from build123d import *

# Parameters (mm, degrees)
SKETCH1_W            = 116.84
SKETCH1_H            = 86.36
BOSS_EXTRUDE2_DEPTH  = 5.08
FILLET1_R            = 12.7
SKETCH3_W            = 116.84
SKETCH3_H            = 60.96
SKETCH3_W_2          = 111.76
SKETCH3_H_2          = 55.88
BOSS_EXTRUDE3_DEPTH  = 38.1
SKETCH4_W            = 10.16
SKETCH4_H            = 10.16
BOSS_EXTRUDE5_DEPTH  = 34.29
FILLET3_R            = 5.08
SKETCH5_R            = 1.27
CUT_EXTRUDE1_DEPTH   = 34.29
CUT_EXTRUDE2_START   = -5.08
SKETCH6_W            = 198.457473549
SKETCH6_H            = 149.814535244
SKETCH6_W_2          = 116.84
SKETCH6_H_2          = 60.96
CUT_EXTRUDE2_DEPTH   = 5.08
FILLET6_R            = 5.08
CUT_EXTRUDE3_REACH   = 146.713
SKETCH7_R            = 12.7
SKETCH7_R_2          = 2.159
CUT_EXTRUDE4_REACH   = 146.713
SKETCH8_R            = 3.175
BOSS_EXTRUDE9_DEPTH  = 5.08
SKETCH14_R           = 1.27
CUT_EXTRUDE6_DEPTH   = 8.89
SKETCH21_W           = 111.76
SKETCH21_H           = 55.88
CUT_EXTRUDE7_DEPTH   = 29.21
SKETCH22_W           = 20.924478465
SKETCH22_H           = 12.476012494
SKETCH22_W_2         = 15.618152649
SKETCH22_H_2         = 14.190033702
SKETCH22_W_3         = 16.110334819
SKETCH22_H_3         = 13.876033943
SKETCH22_W_4         = 12.045494613
CUT_EXTRUDE8_DEPTH   = 5.08
FILLET7_R            = 2.54
BOSS_EXTRUDE10_DEPTH = 5.08


with BuildPart() as part:
    # Sketch1 → Boss-Extrude2 (new body)
    with BuildSketch(Plane(origin=(0, 0, 0), x_dir=(1, 0, 0), z_dir=(0, 1, 0))):
        with Locations((58.42, 43.18)):
            Rectangle(SKETCH1_W, SKETCH1_H)
    extrude(amount=BOSS_EXTRUDE2_DEPTH)

    # Fillet1
    fillet1_edges = [part.edges().sort_by_distance(p)[0] for p in [
        (0, 2.54, -86.36),
        (116.84, 2.54, -86.36),
        (116.84, 2.54, 0),
        (0, 2.54, 0),
    ]]
    fillet(fillet1_edges, radius=FILLET1_R)

    # Sketch3 → Boss-Extrude3 (add)
    with BuildSketch(Plane(origin=(0, 5.08, 0), x_dir=(1, 0, 0), z_dir=(0, 1, 0))):
        with Locations((58.42, 43.18)):
            Rectangle(SKETCH3_W, SKETCH3_H)
        with Locations((58.42, 43.18)):
            Rectangle(SKETCH3_W_2, SKETCH3_H_2, mode=Mode.SUBTRACT)
    extrude(amount=BOSS_EXTRUDE3_DEPTH)

    # Sketch4 → Boss-Extrude5 (add)
    with BuildSketch(Plane(origin=(0, 5.08, 0), x_dir=(1, 0, 0), z_dir=(0, 1, 0))):
        with Locations((7.62, 66.04)):
            Rectangle(SKETCH4_W, SKETCH4_H)
        with Locations((109.22, 66.04)):
            Rectangle(SKETCH4_W, SKETCH4_H)
        with Locations((109.22, 20.32)):
            Rectangle(SKETCH4_W, SKETCH4_H)
        with Locations((7.62, 20.32)):
            Rectangle(SKETCH4_W, SKETCH4_H)
    extrude(amount=BOSS_EXTRUDE5_DEPTH)

    # Fillet3
    fillet3_edges = [part.edges().sort_by_distance(p)[0] for p in [
        (12.7, 22.225, -25.4),
        (12.7, 22.225, -60.96),
        (104.14, 22.225, -60.96),
        (104.14, 22.225, -25.4),
    ]]
    fillet(fillet3_edges, radius=FILLET3_R)

    # Sketch5 → Cut-Extrude1 (cut)
    with BuildSketch(Plane(origin=(0, 39.37, 0), x_dir=(1, 0, 0), z_dir=(0, 1, 0))):
        with Locations(Location((7.62, 66.04, 0), (0, 0, 270))):
            Circle(SKETCH5_R)
        with Locations(Location((109.22, 66.04, 0), (0, 0, 270))):
            Circle(SKETCH5_R)
        with Locations(Location((109.22, 20.32, 0), (0, 0, 270))):
            Circle(SKETCH5_R)
        with Locations(Location((7.62, 20.32, 0), (0, 0, 270))):
            Circle(SKETCH5_R)
    extrude(amount=-CUT_EXTRUDE1_DEPTH, mode=Mode.SUBTRACT)

    # Sketch6 → Cut-Extrude2 (cut)
    with BuildSketch(Plane(origin=(0, 5.08, 0), x_dir=(1, 0, 0), z_dir=(0, 1, 0)).offset(CUT_EXTRUDE2_START)):
        with Locations((67.603582621, 44.619641428)):
            Rectangle(SKETCH6_W, SKETCH6_H)
        with Locations((58.42, 43.18)):
            Rectangle(SKETCH6_W_2, SKETCH6_H_2, mode=Mode.SUBTRACT)
    extrude(amount=CUT_EXTRUDE2_DEPTH, mode=Mode.SUBTRACT)

    # Fillet6
    fillet6_edges = [part.edges().sort_by_distance(p)[0] for p in [
        (0, 21.59, -12.7),
        (0, 21.59, -73.66),
        (116.84, 21.59, -12.7),
        (116.84, 21.59, -73.66),
    ]]
    fillet(fillet6_edges, radius=FILLET6_R)

    # Sketch7 → Cut-Extrude3 (cut, up to next)
    with BuildSketch(Plane(origin=(116.84, 0, 0), x_dir=(0, 0, -1), z_dir=(1, 0, 0)), mode=Mode.PRIVATE) as cut_extrude3_sk1:
        with Locations((43.18, 24.13)):
            Circle(SKETCH7_R)
    cut_extrude3_tool1 = extrude(cut_extrude3_sk1.sketch, amount=-CUT_EXTRUDE3_REACH, mode=Mode.PRIVATE) & part.part
    # Sketch7 → Cut-Extrude3 (cut, up to next)
    with BuildSketch(Plane(origin=(116.84, 0, 0), x_dir=(0, 0, -1), z_dir=(1, 0, 0)), mode=Mode.PRIVATE) as cut_extrude3_sk2:
        with Locations((28.0035, 35.3568)):
            Circle(SKETCH7_R_2)
    cut_extrude3_tool2 = extrude(cut_extrude3_sk2.sketch, amount=-CUT_EXTRUDE3_REACH, mode=Mode.PRIVATE) & part.part
    # Sketch7 → Cut-Extrude3 (cut, up to next)
    with BuildSketch(Plane(origin=(116.84, 0, 0), x_dir=(0, 0, -1), z_dir=(1, 0, 0)), mode=Mode.PRIVATE) as cut_extrude3_sk3:
        with Locations((58.3565, 35.3568)):
            Circle(SKETCH7_R_2)
    cut_extrude3_tool3 = extrude(cut_extrude3_sk3.sketch, amount=-CUT_EXTRUDE3_REACH, mode=Mode.PRIVATE) & part.part
    # Sketch7 → Cut-Extrude3 (cut, up to next)
    with BuildSketch(Plane(origin=(116.84, 0, 0), x_dir=(0, 0, -1), z_dir=(1, 0, 0)), mode=Mode.PRIVATE) as cut_extrude3_sk4:
        with Locations((28.0035, 12.9032)):
            Circle(SKETCH7_R_2)
    cut_extrude3_tool4 = extrude(cut_extrude3_sk4.sketch, amount=-CUT_EXTRUDE3_REACH, mode=Mode.PRIVATE) & part.part
    # Sketch7 → Cut-Extrude3 (cut, up to next)
    with BuildSketch(Plane(origin=(116.84, 0, 0), x_dir=(0, 0, -1), z_dir=(1, 0, 0)), mode=Mode.PRIVATE) as cut_extrude3_sk5:
        with Locations((58.3565, 12.9032)):
            Circle(SKETCH7_R_2)
    cut_extrude3_tool5 = extrude(cut_extrude3_sk5.sketch, amount=-CUT_EXTRUDE3_REACH, mode=Mode.PRIVATE) & part.part
    add(cut_extrude3_tool1.solids().sort_by_distance((116.84, 24.13, -43.18))[0], mode=Mode.SUBTRACT)
    add(cut_extrude3_tool2.solids().sort_by_distance((116.84, 35.3568, -28.0035))[0], mode=Mode.SUBTRACT)
    add(cut_extrude3_tool3.solids().sort_by_distance((116.84, 35.3568, -58.3565))[0], mode=Mode.SUBTRACT)
    add(cut_extrude3_tool4.solids().sort_by_distance((116.84, 12.9032, -28.0035))[0], mode=Mode.SUBTRACT)
    add(cut_extrude3_tool5.solids().sort_by_distance((116.84, 12.9032, -58.3565))[0], mode=Mode.SUBTRACT)

    # Sketch8 → Cut-Extrude4 (cut, up to next)
    with BuildSketch(Plane.ZY, mode=Mode.PRIVATE) as cut_extrude4_sk1:
        with Locations((-43.18, 10.16)):
            Circle(SKETCH8_R)
    cut_extrude4_tool1 = extrude(cut_extrude4_sk1.sketch, amount=-CUT_EXTRUDE4_REACH, mode=Mode.PRIVATE) & part.part
    add(cut_extrude4_tool1.solids().sort_by_distance((0, 10.16, -43.18))[0], mode=Mode.SUBTRACT)

    # Sketch10 → Boss-Extrude9 (add)
    with BuildSketch(Plane(origin=(0, 5.08, 0), x_dir=(1, 0, 0), z_dir=(0, 1, 0))):
        with BuildLine():
            Line((69.85, 19.05), (69.85, 15.24))
            Line((69.85, 15.24), (64.77, 15.24))
            Line((64.77, 15.24), (64.77, 19.05))
            ThreePointArc((64.77, 19.05), (67.31, 21.59), (69.85, 19.05))
        make_face()
        with BuildLine():
            Line((71.12, 67.31), (71.12, 71.12))
            Line((71.12, 71.12), (66.04, 71.12))
            Line((66.04, 71.12), (66.04, 67.31))
            ThreePointArc((66.04, 67.31), (68.58, 64.77), (71.12, 67.31))
        make_face()
    extrude(amount=BOSS_EXTRUDE9_DEPTH)

    # Sketch14 → Cut-Extrude6 (cut)
    with BuildSketch(Plane(origin=(0, 10.16, 0), x_dir=(1, 0, 0), z_dir=(0, 1, 0))):
        with Locations(Location((67.31, 19.05, 0), (0, 0, 270))):
            Circle(SKETCH14_R)
        with Locations(Location((68.58, 67.31, 0), (0, 0, 270))):
            Circle(SKETCH14_R)
    extrude(amount=-CUT_EXTRUDE6_DEPTH, mode=Mode.SUBTRACT)

    # Sketch21 → Cut-Extrude7 (cut)
    with BuildSketch(Plane(origin=(0, 39.37, 0), x_dir=(1, 0, 0), z_dir=(0, 1, 0))):
        with Locations((58.42, 43.18)):
            Rectangle(SKETCH21_W, SKETCH21_H)
    extrude(amount=-CUT_EXTRUDE7_DEPTH, mode=Mode.SUBTRACT)

    # Sketch22 → Cut-Extrude8 (cut)
    with BuildSketch(Plane(origin=(0, 10.16, 0), x_dir=(1, 0, 0), z_dir=(0, 1, 0))):
        with Locations((103.837760768, 21.478006247)):
            Rectangle(SKETCH22_W, SKETCH22_H)
        with Locations((106.490923675, 64.024983149)):
            Rectangle(SKETCH22_W_2, SKETCH22_H_2)
        with Locations((10.59516741, 22.178016971)):
            Rectangle(SKETCH22_W_3, SKETCH22_H_3)
        with Locations((8.562747307, 64.024983149)):
            Rectangle(SKETCH22_W_4, SKETCH22_H_2)
    extrude(amount=-CUT_EXTRUDE8_DEPTH, mode=Mode.SUBTRACT)

    # Fillet7
    fillet7_edges = [part.edges().sort_by_distance(p)[0] for p in [
        (2.54, 24.13, -15.24),
        (114.3, 24.13, -15.24),
        (114.3, 24.13, -71.12),
        (2.54, 24.13, -71.12),
    ]]
    fillet(fillet7_edges, radius=FILLET7_R)

    # Sketch15 → Boss-Extrude10 (add)
    with BuildSketch(Plane(origin=(0, 5.08, 0), x_dir=(1, 0, 0), z_dir=(0, 1, 0))):
        with BuildLine():
            Line((21.59, 33.02), (21.59, 35.56))
            ThreePointArc((21.59, 35.56), (26.67, 40.64), (31.75, 35.56))
            Line((31.75, 35.56), (31.75, 33.02))
            ThreePointArc((31.75, 33.02), (26.67, 27.94), (21.59, 33.02))
        make_face()
    extrude(amount=BOSS_EXTRUDE10_DEPTH)


solid = part.part
Design review of the part built by this model. Coordinates are the model's own, in mm. A direction names the side the tool comes from. Round coordinates to 2 decimals unless told otherwise and drop trailing zeros. Write each loop counter-clockwise with the first axis right and the second up, starting at its lowest first coordinate (ties: lowest second). Pieces come first, ordered by that corner, then holes. Notation, with made-up numbers: (17.5, 29) - (41.5, 29) arc R11 ccw to (41.5, 38) - close; hole circle Ø2 at (-38, 49). An arc over 180 degrees is marked (long way). Use a Markdown table: item, result. Add a question column.
1. We need section C-C (y = 17.5). State the section outline as (x, z) points.
2. We need section D-D (z = -58). State the section outline as (x, y) points.
3. We need section B-B (x = 84). State the section outline as (y, z) points.
4. We need section A-A (z = -43.18). State the section outline as (x, y) points (3 decimals), then the cut area to 3 significant figures.
5. Wall thickness on probe 1 along X at (y, z) = (8.5, -19); probe 2 along Z at (x, y) = (64, 18.5); probe 3 along X at (y, z) = (6, -67): over which ranges is each line inside the solid? List them lowest first.
6. Mouldability with a two-part tool opening along X and no side actions: class faces 1 (the face through (58, 43.18, -14)), 2 (the face through (113.536, 23.863, -70.396)), 3 (the face through (1.528, 21.288, -72.211)) as +X half, -X half, draft (parallel to the pull), parting line (faces both ways), or undercut.
7. Clearance check with flat-ended pins moving along their axes: pin 1 (1.1 mm diameter, centred on y = 7, z = -70, fed in from -X); pin 2 (7 mm diameter, centred on y = 35.36, z = -28, fed in from +X); pin 3 (1.3 mm diameter, centred on x = 67, z = -19, fed in from +Y); pin 4 (5.5 mm diameter, centred on x = 67.5, z = -19.5, fed in from +Y). State where each tip first meets the part, or that it passes through.
8. For faces 4 (the face through (115.6, 13, -56.2)), 5 (the face through (114.3, 11, -43)), 6 (the face through (1.528, 21.892, -14.149)), list the 3-axis set-ups (+Z, -Z, +X, -X, +Y, -Y) from which the entire face can be reached by the end or side of a thin tool; tool diameter is ignored.
Output:
| question | item | result |
|---|---|---|
| 1 | outline | (0, -68.58) arc R5.08 ccw to (5.08, -73.66) - (111.76, -73.66) arc R5.08 ccw to (116.84, -68.58) - (116.84, -54.01) - (114.3, -54.01) - (114.3, -68.58) arc R2.54 cw to (111.76, -71.12) - (5.08, -71.12) arc R2.54 cw to (2.54, -68.58) - (2.54, -17.78) arc R2.54 cw to (5.08, -15.24) - (111.76, -15.24) arc R2.54 cw to (114.3, -17.78) - (114.3, -32.35) - (116.84, -32.35) - (116.84, -17.78) arc R5.08 ccw to (111.76, -12.7) - (5.08, -12.7) arc R5.08 ccw to (0, -17.78) - close |
| 2 | outline | (0, 0) - (116.84, 0) - (116.84, 10.77) - (114.3, 10.77) - (114.3, 5.08) - (2.54, 5.08) - (2.54, 43.18) - (0, 43.18) - close; (114.3, 15.03) - (116.84, 15.03) - (116.84, 33.23) - (114.3, 33.23) - close; (114.3, 37.49) - (116.84, 37.49) - (116.84, 43.18) - (114.3, 43.18) - close |
| 3 | outline | (0, -73.66) - (43.18, -73.66) - (43.18, -71.12) - (5.08, -71.12) - (5.08, -15.24) - (43.18, -15.24) - (43.18, -12.7) - (0, -12.7) - close |
| 4 | outline | (0, 0) - (116.84, 0) - (116.84, 11.43) - (114.3, 11.43) - (114.3, 5.08) - (2.54, 5.08) - (2.54, 6.985) - (0, 6.985) - close; (0, 13.335) - (2.54, 13.335) - (2.54, 43.18) - (0, 43.18) - close; (114.3, 36.83) - (116.84, 36.83) - (116.84, 43.18) - (114.3, 43.18) - close |
| 4 | area | 706 mm2 |
| 5 | probe 1 | x = 0 to 2.54, 64.77 to 66.04, 68.58 to 69.85, 114.3 to 116.84 |
| 5 | probe 2 | z = -73.66 to -71.12, -15.24 to -12.7 |
| 5 | probe 3 | x = 0 to 2.54, 66.06 to 67.35, 69.81 to 71.1, 114.3 to 116.84 |
| 6 | face 1 | draft |
| 6 | face 2 | undercut |
| 6 | face 3 | -X half |
| 7 | pin 1 | stops at x = 0.08 |
| 7 | pin 2 | stops at x = 116.84 |
| 7 | pin 3 | stops at y = 1.27 |
| 7 | pin 4 | stops at y = 10.16 |
| 8 | face 4 | +X |
| 8 | face 5 | +Y |
| 8 | face 6 | +Z, -X, +Y, -Y |
